```python
from build123d import *

# Parameters (mm, degrees)
STOCK_DGT_START                               = 19.05
STOCK_DGT_INSIDE_SWERVE_STRUCTURE_SM_2_R      = 1.7272
STOCK_DGT_INSIDE_SWERVE_STRUCTURE_SM_2_R_2    = 1.35255
STOCK_DGT_INSIDE_SWERVE_STRUCTURE_SMALL_DEPTH = 4.7625
SKETCH2_W                                     = 7.792882402
SKETCH2_H                                     = 6.604
CUT_EXTRUDE2_DEPTH                            = 46.013187304
CUT_EXTRUDE1_DEPTH                            = 46.013187304
FILLET1_R                                     = 2.54
FILLET2_R                                     = 2.54
FILLET3_R                                     = 12.7
FILLET4_R                                     = 1.905
FILLET5_R                                     = 0.635


# Read off the part's stored shape, not the designer's step: Stock-DGT inside swerve structure Small Bearing-1
with BuildPart() as part:
    # Stock-DGT inside swerve structure Sm 2 → Stock-DGT inside swerve structure Small Bearing-1 (new body)
    with BuildSketch(Plane(origin=(0, 0, 0), x_dir=(1, 0, 0), z_dir=(0, 1, 0)).offset(STOCK_DGT_START)):
        with BuildLine():
            Line((26.9875, 3.175), (34.780382402, 3.175))
            ThreePointArc((34.780382402, 3.175), (33.784635987, 8.851779269), (31.868840091, 14.2875))
            Line((31.868840091, 14.2875), (30.633697592, 14.2875))
            Line((30.633697592, 14.2875), (18.578944076, 21.181441452))
            ThreePointArc((18.578944076, 21.181441452), (0, 28.175), (-18.578944076, 21.181441452))
            Line((-18.578944076, 21.181441452), (-30.633697592, 14.2875))
            Line((-30.633697592, 14.2875), (-31.868840091, 14.2875))
            ThreePointArc((-31.868840091, 14.2875), (-33.784635987, 8.851779269), (-34.780382402, 3.175))
            Line((-34.780382402, 3.175), (-26.9875, 3.175))
            Line((-26.9875, 3.175), (-26.9875, -3.175))
            Line((-26.9875, -3.175), (-34.780382402, -3.175))
            ThreePointArc((-34.780382402, -3.175), (-33.784635987, -8.851779269), (-31.868840091, -14.2875))
            Line((-31.868840091, -14.2875), (-30.633697592, -14.2875))
            Line((-30.633697592, -14.2875), (-18.578944076, -21.181441452))
            ThreePointArc((-18.578944076, -21.181441452), (0, -28.175), (18.578944076, -21.181441452))
            Line((18.578944076, -21.181441452), (30.633697592, -14.2875))
            Line((30.633697592, -14.2875), (31.868840091, -14.2875))
            ThreePointArc((31.868840091, -14.2875), (33.784635987, -8.851779269), (34.780382402, -3.175))
            Line((34.780382402, -3.175), (26.9875, -3.175))
            Line((26.9875, -3.175), (26.9875, 3.175))
        make_face()
        with Locations((-14.933176064, -16.8275)):
            Circle(STOCK_DGT_INSIDE_SWERVE_STRUCTURE_SM_2_R, mode=Mode.SUBTRACT)
        with Locations((-30.1625, -11.1125)):
            Circle(STOCK_DGT_INSIDE_SWERVE_STRUCTURE_SM_2_R_2, mode=Mode.SUBTRACT)
        with Locations((14.933176064, -16.8275)):
            Circle(STOCK_DGT_INSIDE_SWERVE_STRUCTURE_SM_2_R, mode=Mode.SUBTRACT)
        with Locations((30.1625, -11.1125)):
            Circle(STOCK_DGT_INSIDE_SWERVE_STRUCTURE_SM_2_R_2, mode=Mode.SUBTRACT)
        with Locations((-30.1625, 11.1125)):
            Circle(STOCK_DGT_INSIDE_SWERVE_STRUCTURE_SM_2_R_2, mode=Mode.SUBTRACT)
        with Locations((-14.933176064, 16.8275)):
            Circle(STOCK_DGT_INSIDE_SWERVE_STRUCTURE_SM_2_R, mode=Mode.SUBTRACT)
        with BuildLine():
            Line((22.394471276, -11.1125), (13.879508051, -11.1125))
            ThreePointArc((13.879508051, -11.1125), (12.572358569, -12.572358569), (11.1125, -13.879508051))
            Line((11.1125, -13.879508051), (11.1125, -19.116031394))
            Line((11.1125, -19.116031394), (-11.1125, -19.116031394))
            Line((-11.1125, -19.116031394), (-11.1125, -11.33701763))
            ThreePointArc((-11.1125, -11.33701763), (-11.940671716, -10.461165517), (-12.7, -9.525))
            Line((-12.7, -9.525), (-20.6375, -9.525))
            Line((-20.6375, -9.525), (-20.6375, 9.525))
            Line((-20.6375, 9.525), (-12.7, 9.525))
            ThreePointArc((-12.7, 9.525), (-11.940671716, 10.461165517), (-11.1125, 11.33701763))
            Line((-11.1125, 11.33701763), (-11.1125, 19.116031394))
            Line((-11.1125, 19.116031394), (11.1125, 19.116031394))
            Line((11.1125, 19.116031394), (11.1125, 13.879508051))
            ThreePointArc((11.1125, 13.879508051), (12.572358569, 12.572358569), (13.879508051, 11.1125))
            Line((13.879508051, 11.1125), (22.394471276, 11.1125))
            ThreePointArc((22.394471276, 11.1125), (25, 0), (22.394471276, -11.1125))
        make_face(mode=Mode.SUBTRACT)
        with Locations((30.1625, 11.1125)):
            Circle(STOCK_DGT_INSIDE_SWERVE_STRUCTURE_SM_2_R_2, mode=Mode.SUBTRACT)
        with Locations((14.933176064, 16.8275)):
            Circle(STOCK_DGT_INSIDE_SWERVE_STRUCTURE_SM_2_R, mode=Mode.SUBTRACT)
    extrude(amount=STOCK_DGT_INSIDE_SWERVE_STRUCTURE_SMALL_DEPTH)

    # Sketch2 → Cut-Extrude2 (cut, through all)
    with BuildSketch(Plane(origin=(0, 23.8125, 0), x_dir=(1, 0, 0), z_dir=(0, 1, 0))):
        with Locations((-30.883941201, 0)):
            Rectangle(SKETCH2_W, SKETCH2_H)
    cut_extrude2 = extrude(amount=-CUT_EXTRUDE2_DEPTH, mode=Mode.SUBTRACT)

    # Sketch1 → Cut-Extrude1 (cut, through all)
    with BuildSketch(Plane(origin=(0, 23.8125, 0), x_dir=(1, 0, 0), z_dir=(0, 1, 0))):
        with BuildLine():
            Line((-28.2575, -3.302), (-28.2575, 3.302))
            ThreePointArc((-28.2575, 3.302), (-27.6225, 3.937), (-26.9875, 3.302))
            Line((-26.9875, 3.302), (-26.9875, -3.302))
            ThreePointArc((-26.9875, -3.302), (-27.6225, -3.937), (-28.2575, -3.302))
        make_face()
    cut_extrude1 = extrude(amount=-CUT_EXTRUDE1_DEPTH, mode=Mode.SUBTRACT)

    # Mirror1: Cut-Extrude2, Cut-Extrude1 across plane
    add(cut_extrude2.mirror(Plane(origin=(0, 0, 0), x_dir=(0, 0, 1), z_dir=(1, 0, 0))), mode=Mode.SUBTRACT)
    add(cut_extrude1.mirror(Plane(origin=(0, 0, 0), x_dir=(0, 0, 1), z_dir=(1, 0, 0))), mode=Mode.SUBTRACT)

    # Fillet1
    fillet1_edges = [part.edges().sort_by_distance(p)[0] for p in [
        (-28.2575, 21.43125, 3.302),
        (-28.2575, 21.43125, -3.302),
        (28.2575, 21.43125, 3.302),
        (28.2575, 21.43125, -3.302),
    ]]
    fillet(fillet1_edges, radius=FILLET1_R)

    # Fillet2
    # the kernel refuses this fillet: 2.54 mm, written as the material it takes off along each edge
    with BuildSketch(Plane(origin=(31.868840091, 14.791233758, -14.2875), x_dir=(-1, 0, 0), z_dir=(0, 1, 0))) as fillet2_piece_1:
        with BuildLine():
            CenterArc((1.70687253, 2.495810645), FILLET2_R, 201.352796162, 57.94406273)
            Line((-0.658771985, 1.570972265), (-0.706084875, 1.552475497))
            ThreePointArc((-0.706084875, 1.552475497), (-0.385813379, 0.761823855), (-0.046354676, -0.020781818))
            Line((-0.046354676, -0.020781818), (0, -0.0508))
            ThreePointArc((0, -0.0508), (0.61757125, -0.0508), (1.225707898, -0.049916213))
            Line((1.225707898, -0.049916213), (1.235142499, 0))
        make_face()
    extrude(amount=13.280032484, mode=Mode.SUBTRACT)
    with BuildSketch(Plane(origin=(31.868840091, 14.791233758, 14.2875), x_dir=(-1, 0, 0), z_dir=(0, 1, 0))) as fillet2_piece_2:
        with BuildLine():
            CenterArc((1.70687253, -2.495810645), FILLET2_R, 100.703141108, 57.94406273)
            Line((-0.658771985, -1.570972265), (-0.706084875, -1.552475497))
            ThreePointArc((-0.706084875, -1.552475497), (-0.385813379, -0.761823855), (-0.046354676, 0.020781818))
            Line((-0.046354676, 0.020781818), (0, 0.0508))
            ThreePointArc((0, 0.0508), (0.61757125, 0.0508), (1.225707898, 0.049916213))
            Line((1.225707898, 0.049916213), (1.235142499, 0))
        make_face()
    extrude(amount=13.280032484, mode=Mode.SUBTRACT)
    with BuildSketch(Plane(origin=(-31.868840091, 14.791233758, 14.2875), x_dir=(-0.3867152758408876, 0, -0.9221991625626789), z_dir=(0, 1, 0))) as fillet2_piece_3:
        with BuildLine():
            CenterArc((1.641560806, -2.53924452), FILLET2_R, 88.602528123, 57.94406273)
            Line((-0.477648472, -1.139047378), (-0.520032658, -1.111043435))
            ThreePointArc((-0.520032658, -1.111043435), (-0.285671954, -0.549878553), (-0.046847717, 0.019645136))
            Line((-0.046847717, 0.019645136), (-0.001238914, 0.05078489))
            ThreePointArc((-0.001238914, 0.05078489), (0.851753248, 0.061187853), (1.704745411, 0.05078489))
            Line((1.704745411, 0.05078489), (1.703506497, 0))
        make_face()
    extrude(amount=13.280032484, mode=Mode.SUBTRACT)
    with BuildSketch(Plane(origin=(-31.868840091, 14.791233758, -14.2875), x_dir=(-0.3867152758408886, 0, 0.9221991625626784), z_dir=(0, 1, 0))) as fillet2_piece_4:
        with BuildLine():
            CenterArc((1.641560806, 2.53924452), FILLET2_R, 213.453409147, 57.94406273)
            Line((-0.477648472, 1.139047378), (-0.520032658, 1.111043435))
            ThreePointArc((-0.520032658, 1.111043435), (-0.285671954, 0.549878553), (-0.046847717, -0.019645136))
            Line((-0.046847717, -0.019645136), (-0.001238914, -0.05078489))
            ThreePointArc((-0.001238914, -0.05078489), (0.851753248, -0.061187853), (1.704745411, -0.05078489))
            Line((1.704745411, -0.05078489), (1.703506497, 0))
        make_face()
    extrude(amount=13.280032484, mode=Mode.SUBTRACT)

    # Fillet3
    fillet3_edges = [part.edges().sort_by_distance(p)[0] for p in [
        (-18.578944076, 21.43125, -21.181441452),
        (18.578944076, 21.43125, -21.181441452),
        (30.633697592, 21.43125, -14.2875),
        (-30.633697592, 21.43125, -14.2875),
        (30.633697592, 21.43125, 14.2875),
        (-18.578944076, 21.43125, 21.181441452),
        (18.578944076, 21.43125, 21.181441452),
        (-30.633697592, 21.43125, 14.2875),
    ]]
    fillet(fillet3_edges, radius=FILLET3_R)

    # Fillet4
    fillet4_edges = [part.edges().sort_by_distance(p)[0] for p in [
        (11.1125, 21.43125, 19.116031394),
        (-11.1125, 21.43125, -19.116031394),
        (11.1125, 21.43125, -19.116031394),
        (-11.1125, 21.43125, 19.116031394),
        (-12.7, 21.43125, -9.525),
        (-12.7, 21.43125, 9.525),
        (-20.6375, 21.43125, 9.525),
        (-20.6375, 21.43125, -9.525),
        (22.394471276, 21.43125, 11.1125),
        (22.394471276, 21.43125, -11.1125),
        (11.1125, 21.43125, -13.879508051),
        (11.1125, 21.43125, 13.879508051),
        (13.879508051, 21.43125, 11.1125),
        (13.879508051, 21.43125, -11.1125),
        (-11.1125, 21.43125, 11.33701763),
        (-11.1125, 21.43125, -11.33701763),
    ]]
    fillet(fillet4_edges, radius=FILLET4_R)

    # Fillet5
    fillet5_edges = [part.edges().sort_by_distance(p)[0] for p in [
        (-34.768555061, 21.43125, 3.302),
        (-34.768555061, 21.43125, -3.302),
        (34.768555061, 21.43125, 3.302),
        (34.768555061, 21.43125, -3.302),
    ]]
    fillet(fillet5_edges, radius=FILLET5_R)


solid = part.part
```
CAD build for the part. Positions are in the model's coordinates, mm. A direction names the side the tool comes from. Coordinates: 2 decimals unless noted, no trailing zeros. Loops run counter-clockwise (first coordinate to the right, second up) from the corner with the lowest first, then second, coordinate; pieces in that order, holes last. Notation, with made-up numbers: (39.5, 68) - (70.5, 68) arc R25 cw to (70.5, 99) - close; hole circle Ø6 at (69.5, 38). An arc over 180 degrees is marked (long way). Use CSV: the item, a comma, the result in double quotes. Start each with the question number.
Q1. Drop flat-ended pins along their axis: P1, Ø3, axis at x = 14.93, z = 16.83, coming from the -Y side; P2, Ø2, axis at y = 21, z = 15.5, coming from the -X side; P3, Ø1.4, axis at x = 18.5, y = 21, coming from the -Z side; P4, Ø1.4, axis at x = -32.5, y = 20.5, coming from the +Z side. Give the stop position or say it passes through.
Q2. Probe probe 1 along Z at (x, y) = (-15, 23.5) (3 decimals); probe 2 along X at (y, z) = (20.35, 15.5); probe 3 along X at (y, z) = (21.95, -11.5). List the from-to ranges inside material, lowest first. Write a range as from..to.
Q3. Cut at C-C, the plane y = 21.45. State how many separate pieces and enclosed holes the cut face has, then the cut area to 3 significant figures.
Q4. 3-axis set-ups, long thin cutter, end or side, ignore diameter. For faces 1 (the cylindrical face through (-30.34, 21.46, -14.49)), 2 (the flat face through (-16, 21, -9.525)), 3 (the flat face through (-32, 21, -3.302)): which of +Z, -Z, +X, -X, +Y, -Y reach the whole face in a straight line?
Q5. Two-plate mould, pull along X, no slides. Class faces 4 (the cylindrical face through (-33.876, 21.398, -8.494)), 5 (the flat face through (26.988, 21, 0)), 6 (the cylindrical face through (-20.065, 21.465, 8.982)): +X half, -X half, draft (parallel to the pull), parting line (faces both ways), or undercut.
Q6. Cut at B-B, the plane z = -23. List the corners of the cut face in (x, y), then the cut area to 3 significant figures.
Q7. Cut at A-A, the plane z = -1. List the corners of the cut face in (x, y), then the cut area to 3 significant figures.
Here are the results:
1,P1,"through"
1,P2,"x = -30.32"
1,P3,"z = -21.84"
1,P4,"z = 13.73"
2,probe 1,"-23.85..-18.553, -15.102..-9.525, 9.525..15.102, 18.553..23.85"
2,probe 2,"-28.51..-16.04, -13.83..-11.11, 11.11..13.83, 16.04..28.51"
2,probe 3,"-32.98..-31.46, -28.87..-11.21, 13.61..28.87, 31.46..32.98"
3,separate pieces,"1"
3,enclosed holes,"9"
3,area,"1,480 mm2"
4,face 1,"-Z, -X, +Y, -Y"
4,face 2,"+Y, -Y"
4,face 3,"-X, +Y, -Y"
5,face 4,"-X half"
5,face 5,"+X half"
5,face 6,"undercut"
6,outline,"(-16.27, 19.05) - (16.27, 19.05) - (16.27, 23.81) - (-16.27, 23.81) - close"
6,area,"155 mm2"
7,outline,"(-26.99, 19.05) - (-20.64, 19.05) - (-20.64, 23.81) - (-26.99, 23.81) - close; (24.98, 19.05) - (26.99, 19.05) - (26.99, 23.81) - (24.98, 23.81) - close"
7,area,"39.8 mm2"
